Verification items for the finished model (mm, model axes). Give positions to 0.01 mm unless a question says otherwise; leave off trailing zeros. Order: outer loops, then holes, each group sorted by start corner. A loop starts at its lowest first (then second) coordinate and runs counter-clockwise, first axis right, second up.
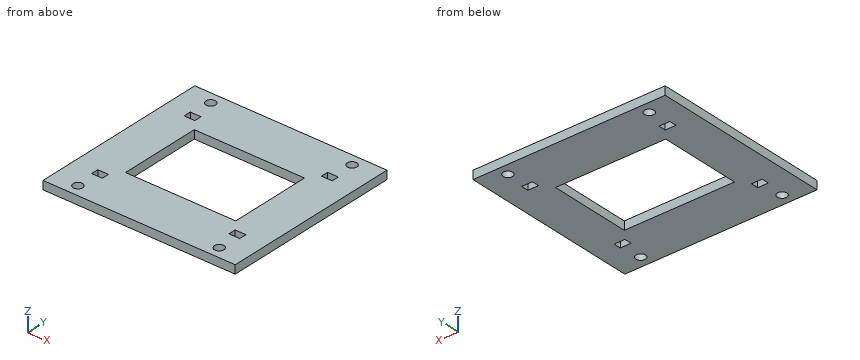
from build123d import *

# Parameters (mm, degrees)
SKETCH_1_W                         = 68
SKETCH_1_H                         = 64
BOARD_MOUNT_BASE_DEPTH             = 3
SOLDER_AND_CONNECTOR_OPENING_START = -0.1
SKETCH_2_W                         = 39
SKETCH_2_H                         = 29
SOLDER_AND_CONNECTOR_OPENING_DEPTH = 3.2
PCB_M2_SLOTS_CENTRES48P6X39_START  = -0.1
SKETCH_3_W                         = 3.8
SKETCH_3_H                         = 2.6
PCB_M2_SLOTS_CENTRES48P6X39_DEPTH  = 3.2
DECK_ATTACHMENT_M3_START           = -0.1
SKETCH_4_R                         = 1.7
DECK_ATTACHMENT_M3_DEPTH           = 3.2


with BuildPart() as part:
    # 草图1 → Board_mount_base (new body)
    with BuildSketch(Plane.XY):
        Rectangle(SKETCH_1_W, SKETCH_1_H)
    extrude(amount=BOARD_MOUNT_BASE_DEPTH)

    # 草图2 → Solder_and_connector_opening (cut)
    with BuildSketch(Plane.XY.offset(SOLDER_AND_CONNECTOR_OPENING_START)):
        Rectangle(SKETCH_2_W, SKETCH_2_H)
    extrude(amount=SOLDER_AND_CONNECTOR_OPENING_DEPTH, mode=Mode.SUBTRACT)

    # 草图3 → PCB_M2_slots_centres48p6x39 (cut)
    with BuildSketch(Plane.XY.offset(PCB_M2_SLOTS_CENTRES48P6X39_START)):
        with Locations((-24.3, -19.5)):
            Rectangle(SKETCH_3_W, SKETCH_3_H)
        with Locations((-24.3, 19.5)):
            Rectangle(SKETCH_3_W, SKETCH_3_H)
        with Locations((24.3, -19.5)):
            Rectangle(SKETCH_3_W, SKETCH_3_H)
        with Locations((24.3, 19.5)):
            Rectangle(SKETCH_3_W, SKETCH_3_H)
    extrude(amount=PCB_M2_SLOTS_CENTRES48P6X39_DEPTH, mode=Mode.SUBTRACT)

    # 草图4 → Deck_attachment_M3 (cut)
    with BuildSketch(Plane.XY.offset(DECK_ATTACHMENT_M3_START)):
        with Locations((-25, -28)):
            Circle(SKETCH_4_R)
        with Locations((-25, 28)):
            Circle(SKETCH_4_R)
        with Locations((25, -28)):
            Circle(SKETCH_4_R)
        with Locations((25, 28)):
            Circle(SKETCH_4_R)
    extrude(amount=DECK_ATTACHMENT_M3_DEPTH, mode=Mode.SUBTRACT)


solid = part.part
(1) Section check D-D, the plane z = 1.45. Give the number of separate pieces and of enclosed holes in the cut face, then the cut area to 3 significant figures.
Solved:
separate pieces: 1
enclosed holes: 9
area: 3,150 mm2
(2) Go/stop test with a flat-tipped pin: pin 1 (2 mm diameter, centred on x = -25, y = 28, fed in from +Z). Record where the tip stops, or that it passes through.
Solved:
pin 1: passes through
(3) Section check C-C, the plane x = 18. Enter the section's corners in (y, z), then the cut area to 3 significant figures.
Solved:
outline: (-32, 0) - (-14.5, 0) - (-14.5, 3) - (-32, 3) - close; (14.5, 0) - (32, 0) - (32, 3) - (14.5, 3) - close
area: 105 mm2
(4) Section check B-B, the plane x = -25. Enter the section's corners in (y, z), then the cut area to 3 significant figures.
Solved:
outline: (-32, 0) - (-29.7, 0) - (-29.7, 3) - (-32, 3) - close; (-26.3, 0) - (-20.8, 0) - (-20.8, 3) - (-26.3, 3) - close; (-18.2, 0) - (18.2, 0) - (18.2, 3) - (-18.2, 3) - close; (20.8, 0) - (26.3, 0) - (26.3, 3) - (20.8, 3) - close; (29.7, 0) - (32, 0) - (32, 3) - (29.7, 3) - close
area: 156 mm2
(5) Scan lines: line 1 (X direction, y = 28, z = 0.85); line 2 (Y direction, x = -25, z = 1); line 3 (Y direction, x = -23, z = 1.25). Record each from-to range of solid material in increasing order.
Solved:
line 1: x = -34 to -26.7, -23.3 to 23.3, 26.7 to 34
line 2: y = -32 to -29.7, -26.3 to -20.8, -18.2 to 18.2, 20.8 to 26.3, 29.7 to 32
line 3: y = -32 to -20.8, -18.2 to 18.2, 20.8 to 32
(6) Section check A-A, the plane y = -28. Enter the section's corners in (x, z).
Solved:
outline: (-34, 0) - (-26.7, 0) - (-26.7, 3) - (-34, 3) - close; (-23.3, 0) - (23.3, 0) - (23.3, 3) - (-23.3, 3) - close; (26.7, 0) - (34, 0) - (34, 3) - (26.7, 3) - close
